For this review, take the finished solid that the model builds, in its own axes (mm). Face numbers are marked on the shaded views. A direction names the side the tool comes from. Coordinates: 2 decimals unless noted, no trailing zeros. Write each loop counter-clockwise with the first axis right and the second up, starting at its lowest first coordinate (ties: lowest second). Pieces come first, ordered by that corner, then holes.
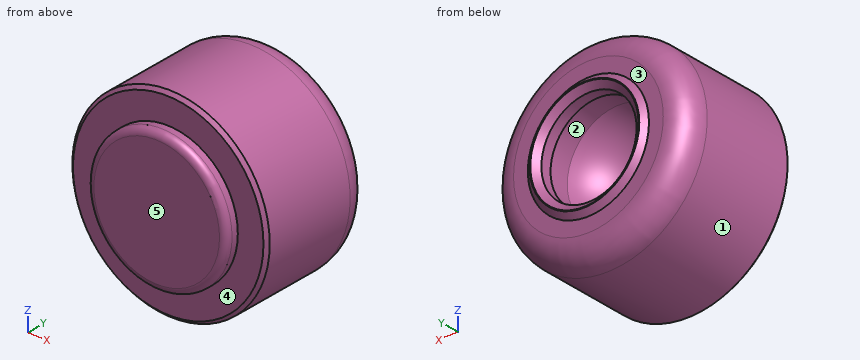
```python
from build123d import *

# Parameters (mm, degrees)
SKETCH2_R                      = 8.9
BOSS_EXTRUDE1_DEPTH            = 0.7
BOSS_EXTRUDE1_TAPER            = 50
F_14_0_14_DIAMETER_HOLE1_D     = 14
F_14_0_14_DIAMETER_HOLE1_DEPTH = 2.4
SKETCH5_R                      = 10.232050808
BOSS_EXTRUDE2_DEPTH            = 2
CHAMFER1_SIZE                  = 0.5
CHAMFER2_SIZE                  = 0.953402874
CHAMFER2_SIZE2                 = 0.8
FILLET1_R                      = 1
FILLET2_R                      = 3.5


with BuildPart() as part:
    # Cut-Extrude1: read off the stored shape, not the designer's step
    # Cut-Extrude1 outline → Cut-Extrude1 (revolve)
    with BuildSketch(Plane.XY):
        with BuildLine():
            Line((0, 10.6), (0, 3))
            Line((0, 3), (14.5, 3))
            Line((14.5, 3), (14.5, 21))
            Line((14.5, 21), (0, 21))
            Line((0, 21), (0, 19.3))
            Line((0, 19.3), (7.493997598, 19.3))
            Line((7.493997598, 19.3), (7.493997598, 15.8))
            ThreePointArc((7.493997598, 15.8), (4.5607017, 12.02732931), (0, 10.6))
        make_face()
    revolve(axis=Axis((0, 0, 0), (0, 1, 0)))

    # Sketch2 → Boss-Extrude1 (add)
    with BuildSketch(Plane(origin=(0, 21, 0), x_dir=(-1, 0, 0), z_dir=(0, 1, 0))):
        Circle(SKETCH2_R)
    extrude(amount=BOSS_EXTRUDE1_DEPTH, taper=BOSS_EXTRUDE1_TAPER)

    # Ø14.0 (14) Diameter Hole1
    with Locations(Plane.XZ.offset(-19.3)):
        with Locations((0, 0)):
            Hole(F_14_0_14_DIAMETER_HOLE1_D / 2, depth=F_14_0_14_DIAMETER_HOLE1_DEPTH)

    # Sketch5 → Boss-Extrude2 (add)
    with BuildSketch(Plane.XZ.offset(-3)):
        Circle(SKETCH5_R)
    extrude(amount=BOSS_EXTRUDE2_DEPTH)

    # Chamfer1
    chamfer1_edges = [part.edges().sort_by_distance(p)[0] for p in [
        (-14.5, 3, 0),
    ]]
    chamfer(chamfer1_edges, length=CHAMFER1_SIZE)

    # Chamfer2
    chamfer2_edges = [part.edges().sort_by_distance(p)[0] for p in [
        (7, 21.7, 0),
    ]]
    chamfer2_side = [part.faces().sort_by_distance(p)[0] for p in [
        (7.837637988, 21.7, 0),
    ]]
    chamfer(chamfer2_edges, length=CHAMFER2_SIZE, length2=CHAMFER2_SIZE2, reference=chamfer2_side[0])

    # Fillet1
    fillet1_edges = [part.edges().sort_by_distance(p)[0] for p in [
        (-10.232050808, 1, 0),
    ]]
    fillet(fillet1_edges, radius=FILLET1_R)

    # Fillet2
    fillet2_edges = [part.edges().sort_by_distance(p)[0] for p in [
        (-14.5, 21, 0),
    ]]
    fillet(fillet2_edges, radius=FILLET2_R)


solid = part.part
```
Q1. Add section A-A (x = 0). State the section outline as (y, z) points.
Ans:
outline: (1, -9.23) arc R1 ccw to (2, -10.23) - (3, -10.23) - (3, -14) - (3.5, -14.5) - (17.5, -14.5) arc R3.5 ccw to (21, -11) - (21, -8.9) - (21.7, -8.07) - (21.7, -7.95) - (20.9, -7) - (19.3, -7) - (19.3, -7.49) - (15.8, -7.49) arc R8 cw to (15.8, 7.49) - (19.3, 7.49) - (19.3, 7) - (20.9, 7) - (21.7, 7.95) - (21.7, 8.07) - (21, 8.9) - (21, 11) arc R3.5 ccw to (17.5, 14.5) - (3.5, 14.5) - (3, 14) - (3, 10.23) - (2, 10.23) arc R1 ccw to (1, 9.23) - close
Q2. Add section C-C (y = 13.75). State the section outline as (x, z) points.
Ans:
outline: circle Ø29 at (0, 0); hole circle Ø12.72 at (0, 0)
Q3. Draft analysis for pull direction X (two halves, no side actions). For the marked faces 1, 2 and 3, state which applies: +X half, -X half, draft (parallel to the pull), parting line (faces both ways), or undercut.
Ans:
face 1: parting line
face 2: undercut
face 3: draft
Q4. For probe 1 along Y at (x, z) = (0, 9); probe 2 along Z at (x, y) = (0, 19.65); probe 3 along Z at (x, y) = (5.5, 18), list the stretches that pass through material, from the lowest coordinate up.
Ans:
probe 1: y = 1 to 21
probe 2: z = -13.76 to -7, 7 to 13.76
probe 3: z = -13.38 to -5.09, 5.09 to 13.38
Q5. Tool access review of the marked faces 4 and 5: name each direction out of +Z, -Z, +X, -X, +Y, -Y from which nothing blocks a thin tool from reaching the whole face with its end or side.
Ans:
face 4: -Y
face 5: +Z, -Z, +X, -X, -Y
Q6. Clearance check with flat-ended pins moving along their axes: pin 1 Ø12 at (x, y) = (-4.5, 19.5) entering from -Z; pin 2 Ø1 at (x, y) = (10.5, 15) entering from +Z; pin 3 Ø3 at (x, y) = (9, 11) entering from +Z; pin 4 Ø1 at (x, y) = (-1.5, 15) entering from +Z. State where each tip first meets the part, or that it passes through.
Ans:
pin 1: stops at z = -14.5
pin 2: stops at z = 10.5
pin 3: stops at z = 12.41
pin 4: stops at z = 14.47
Q7. Add section B-B (y = 5). State the section outline as (x, z) points, then the cut area to 3 significant figures.
Ans:
outline: circle Ø29 at (0, 0)
area: 661 mm2
